Input: part model. Units: mm. Frame: model coordinates. A direction names the side the tool comes from. Coordinates: 2 decimals unless noted, no trailing zeros. Loops run counter-clockwise (first coordinate to the right, second up) from the corner with the lowest first, then second, coordinate; pieces in that order, holes last.
Item 1: Reachability of faces 1 (the flat face through (3, -3, 9)), 2 (the cylindrical face through (2.17, -9.76, -7.92)), 3 (the flat face through (-5.4, -5.4, 0)) from +Z, -Z, +X, -X, +Y, -Y: full face, straight path, thin tool, end or side. Return the list, or none.
Item 2: Contact query for flat-ended pins moving along their axis: P1, Ø7, axis at x = 0, y = 0, coming from the +Z side; P2, Ø1.5, axis at y = 1.5, z = 3.5, coming from the -X side; P3, Ø3, axis at x = 1.5, z = -3, coming from the -Y side; P4, Ø3, axis at y = -9, z = -11.5, coming from the -X side. Output: stop coordinate, or through.
Item 3: Ray query, line 1 along Z through (x, y) = (4.25, -9.25); line 2 along Y through (x, z) = (0, -7.25); line 3 along Z through (x, y) = (-7, 2.75). Return the intervals inside material, ascending.
Item 4: Section C-C on x = 4.75. Return loops of the section in (y, z), and give its area (3 significant figures).
Item 5: Section B-B on z = 4.75. Return loops of the section in (x, y).
Item 6: Section A-A on x = 0. Return loops of the section in (y, z).
Item 7: Section D-D on y = 5.5. Return loops of the section in (x, z).
```python
from build123d import *
from build123d.topology import SkipClean

# Parameters (mm, degrees)
SKETCH_1_R          = 7
SKETCH_1_R_2        = 4
EXTRUDE_1_DEPTH     = 9
EXTRUDE_START       = 2
SKETCH_2_R          = 12.5
SKETCH_2_R_2        = 4
EXTRUDE_2_DEPTH     = 2
SKETCH_3_R          = 10
EXTRUDE_3_DEPTH     = 12
SKETCH_4_R          = 12.5
EXTRUDE_4_DEPTH     = 2
SKETCH_5_R          = 4
CUT_EXTRUDE_1_DEPTH = 31.618621785


with BuildPart() as part:
    # 草图1 → 拉伸1 (new body)
    with BuildSketch(Plane.XY):
        Circle(SKETCH_1_R)
        Circle(SKETCH_1_R_2, mode=Mode.SUBTRACT)
    extrude(amount=EXTRUDE_1_DEPTH)

    # 草图2 → 拉伸2 (add)
    with SkipClean():  # the faces are left unmerged after this step: merging them gives an invalid solid
        with BuildSketch(Plane(origin=(0, 0, 0), x_dir=(-1, 0, 0), z_dir=(0, 0, -1)).offset(EXTRUDE_START)):
            Circle(SKETCH_2_R)
            Circle(SKETCH_2_R_2, mode=Mode.SUBTRACT)
        extrude(amount=-EXTRUDE_2_DEPTH)

    # 草图3 → 拉伸3 (add)
    with SkipClean():  # the faces are left unmerged after this step: merging them gives an invalid solid
        with BuildSketch(Plane(origin=(0, 0, -2), x_dir=(-1, 0, 0), z_dir=(0, 0, -1))):
            Circle(SKETCH_3_R)
        extrude(amount=EXTRUDE_3_DEPTH)

    # 草图4 → 拉伸4 (add)
    with SkipClean():  # the faces are left unmerged after this step: merging them gives an invalid solid
        with BuildSketch(Plane(origin=(0, 0, -14), x_dir=(-1, 0, 0), z_dir=(0, 0, -1)).offset(EXTRUDE_START)):
            Circle(SKETCH_4_R)
        extrude(amount=-EXTRUDE_4_DEPTH)

    # 草图5 → 切除-拉伸1 (cut, through all)
    with SkipClean():  # the faces are left unmerged after this step: merging them gives an invalid solid
        with BuildSketch(Plane.XY.offset(9)):
            Circle(SKETCH_5_R)
        extrude(amount=-CUT_EXTRUDE_1_DEPTH, mode=Mode.SUBTRACT)


solid = part.part
```
Results found:
1. face 1: +Z, +X, -X, +Y, -Y
1. face 2: none
1. face 3: +Z
2. P1: passes through
2. P2: stops at x = -6.96
2. P3: stops at y = -12.49
2. P4: stops at x = -6.61
3. line 1: z = -16 to -14, -2 to 0
3. line 2: y = -10 to -4, 4 to 10
3. line 3: z = -16 to 0
4. outline: (-11.56, -16) - (11.56, -16) - (11.56, -14) - (8.8, -14) - (8.8, -2) - (11.56, -2) - (11.56, 0) - (5.14, 0) - (5.14, 9) - (-5.14, 9) - (-5.14, 0) - (-11.56, 0) - (-11.56, -2) - (-8.8, -2) - (-8.8, -14) - (-11.56, -14) - close
4. area: 396 mm2
5. outline: circle Ø14 at (0, 0); hole circle Ø8 at (0, 0)
6. outline: (-12.5, -16) - (-4, -16) - (-4, 9) - (-7, 9) - (-7, 0) - (-12.5, 0) - (-12.5, -2) - (-10, -2) - (-10, -14) - (-12.5, -14) - close; (4, -16) - (12.5, -16) - (12.5, -14) - (10, -14) - (10, -2) - (12.5, -2) - (12.5, 0) - (7, 0) - (7, 9) - (4, 9) - close
7. outline: (-11.22, -16) - (11.22, -16) - (11.22, -14) - (8.35, -14) - (8.35, -2) - (11.22, -2) - (11.22, 0) - (4.33, 0) - (4.33, 9) - (-4.33, 9) - (-4.33, 0) - (-11.22, 0) - (-11.22, -2) - (-8.35, -2) - (-8.35, -14) - (-11.22, -14) - close
